Geometry: final body of the model. Coordinates: model frame, mm. A direction names the side the tool comes from. Coordinates: 2 decimals unless noted, no trailing zeros. Order: outer loops, then holes, each group sorted by start corner. A loop starts at its lowest first (then second) coordinate and runs counter-clockwise, first axis right, second up. Notation, with made-up numbers: M 62.25,57.5 L 83.25,57.5 A18 cw 83.25,61.5 Z; hole C 69,-9.5 d7. An arc over 180 degrees is marked long. Write item = value, one per line. Start each with the question number.
```python
from build123d import *

# Parameters (mm, degrees)
ESQUISSE1_W             = 50
ESQUISSE1_H             = 17
BOSS_EXTRU_1_DEPTH      = 35
D_POUILLE2_ANGLE        = -5
COQUE2_T                = -1
CONG_1_R                = 1
ESQUISSE2_R             = 2
ESQUISSE2_R_2           = 1
BOSS_EXTRU_2_DEPTH      = 14.5
ENL_V_MAT_EXTRU_1_REACH = 48.249
ENL_V_MAT_EXTRU_2_REACH = 48.249
ESQUISSE4_R             = 1.5


with BuildPart() as part:
    # Esquisse1 → Boss.-Extru.1 (new body)
    with BuildSketch(Plane.XY):
        with Locations((0, 8.5)):
            Rectangle(ESQUISSE1_W, ESQUISSE1_H)
    extrude(amount=BOSS_EXTRU_1_DEPTH)

    # Dépouille2
    d_pouille2_faces = [part.faces().sort_by_distance(p)[0] for p in [
        (0, 8.5, 0),
        (25, 8.5, 17.5),
        (-25, 8.5, 17.5),
        (0, 8.5, 35),
    ]]
    draft(d_pouille2_faces, Plane(origin=(-25, 0, 35), x_dir=(-1, 0, 0), z_dir=(0, -1, 0)), D_POUILLE2_ANGLE)

    # Coque2
    coque2_openings = [part.faces().sort_by_distance(p)[0] for p in [
        (0, 0, 17.5),
    ]]
    offset(amount=COQUE2_T, openings=coque2_openings, kind=Kind.INTERSECTION)

    # Congé1
    cong_1_edges = [part.edges().sort_by_distance(p)[0] for p in [
        (24.25634636, 8.5, 34.25634636),
        (0, 17, 33.51269272),
        (-23.296270854, 8, 1.703729146),
        (-22.596361546, 16, 17.5),
        (23.296270854, 8, 1.703729146),
        (0, 16, 2.403638454),
        (22.596361546, 16, 17.5),
        (-23.296270854, 8, 33.296270854),
        (23.296270854, 8, 33.296270854),
        (0, 16, 32.596361546),
        (-24.25634636, 8.5, 34.25634636),
        (0, 17, 1.48730728),
        (24.25634636, 8.5, 0.74365364),
        (-24.25634636, 8.5, 0.74365364),
        (-23.51269272, 17, 17.5),
        (23.51269272, 17, 17.5),
    ]]
    fillet(cong_1_edges, radius=CONG_1_R)

    # Esquisse2 → Boss.-Extru.2 (add)
    # profile 1 of 2: a face of its own
    with BuildSketch(Plane(origin=(0, 16, 0), x_dir=(-1, 0, 0), z_dir=(0, -1, 0))):
        with Locations(Location((-19.25, -29.25, 0), (0, 0, 270))):
            Circle(ESQUISSE2_R)
        with Locations(Location((-19.25, -29.25, 0), (0, 0, 270))):
            Circle(ESQUISSE2_R_2, mode=Mode.SUBTRACT)
    # profile 2 of 2: a face of its own
    with BuildSketch(Plane(origin=(0, 16, 0), x_dir=(-1, 0, 0), z_dir=(0, -1, 0))):
        with Locations(Location((19.25, -5.75, 0), (0, 0, 270))):
            Circle(ESQUISSE2_R)
        with Locations(Location((19.25, -5.75, 0), (0, 0, 270))):
            Circle(ESQUISSE2_R_2, mode=Mode.SUBTRACT)
    extrude(amount=BOSS_EXTRU_2_DEPTH)

    # Esquisse3 → Enlèv. mat.-Extru.1 (cut, up to next)
    with BuildSketch(Plane(origin=(0, 0, 0), x_dir=(0, 0, -1), z_dir=(1, 0, 0)), mode=Mode.PRIVATE) as enl_v_mat_extru_1_sk1:
        with BuildLine():
            Line((-20, 5), (-20, -1))
            Line((-20, -1), (-15, -1))
            Line((-15, -1), (-15, 5))
            ThreePointArc((-15, 5), (-17.5, 7.5), (-20, 5))
        make_face()
    enl_v_mat_extru_1_tool1 = extrude(enl_v_mat_extru_1_sk1.sketch, amount=-ENL_V_MAT_EXTRU_1_REACH, mode=Mode.PRIVATE) & part.part
    add(enl_v_mat_extru_1_tool1.solids().sort_by_distance((0, 3.001296, 17.5))[0], mode=Mode.SUBTRACT)

    # Enlèv. mat.-Extru.2: up to this plane
    enl_v_mat_extru_2_end = Plane(origin=(25, 0, 35), z_dir=(0.9961946980917455, 0.08715574274765836, 0))
    # Esquisse4 → Enlèv. mat.-Extru.2 (cut, up to the surface)
    with BuildSketch(Plane(origin=(0, 0, 0), x_dir=(0, 0, -1), z_dir=(1, 0, 0)), mode=Mode.PRIVATE) as enl_v_mat_extru_2_sk1:
        with Locations(Location((-8, 6, 0), (0, 0, 90))):
            Circle(ESQUISSE4_R)
    enl_v_mat_extru_2_tool1 = split(extrude(enl_v_mat_extru_2_sk1.sketch, amount=ENL_V_MAT_EXTRU_2_REACH, mode=Mode.PRIVATE), bisect_by=enl_v_mat_extru_2_end, keep=Keep.BOTH, mode=Mode.PRIVATE)
    add(enl_v_mat_extru_2_tool1.solids().sort_by_distance((0, 6, 8))[0], mode=Mode.SUBTRACT)


solid = part.part
```
Item 1: First-contact query: pin 1 (10 mm diameter, centred on x = 2, y = 15, fed in from +Z); pin 2 (10 mm diameter, centred on x = 17.5, y = 8.5, fed in from +Z); pin 3 (4 mm diameter, centred on y = 12, z = 31, fed in from -X). Flat tips, straight axial feed; report the tip coordinate or a pass-through.
Item 2: Reachability of faces 1 (the flat face through (23.345, 7.438, 17.283)), 2 (the cylindrical face through (0.316, 16.744, 33.264)), 3 (the cylindrical face through (-23.9, 7.5, 17.4)) from +Z, -Z, +X, -X, +Y, -Y: full face, straight path, thin tool, end or side. Return the list, or none.
Item 3: Section query B-B on x = 19.25. Output: boundary loops of the cut face in (y, z), and give its area (3 significant figures).
Item 4: Draft query along Z for faces 4 (the cylindrical face through (-24, 8.17, 33.99)), 5 (the cylindrical face through (0.316, 16.744, 1.736)), 6 (the flat face through (20, 1.5, 28)), 7 (the flat face through (-24.306, 7.931, 17.269)). Return one class per face: pulls with the +Z half, pulls with the -Z half, needs draft (parallel to the pull), parting line crosses it, or undercut.
Item 5: Section query A-A on z = 22.5. Output: boundary loops of the cut face in (x, y), and give its area (3 significant figures).
Item 6: Material intervals for probe 1 along Z at (x, y) = (18.5, 14.25); probe 2 along X at (y, z) = (7, 29.25); probe 3 along X at (y, z) = (2.75, 4.5), sorted ascending. Write a range as [from, to].
Item 7: Section query D-D on x = 6.5. Output: boundary loops of the cut face in (y, z), and give its area (3 significant figures).
Item 8: Section query C-C on y = 12.5. Give the number of separate pieces and of enclosed holes in the cut face, and give its area (3 significant figures).
Ans:
q1.pin_1 = 34.13
q1.pin_2 = 34.69
q1.pin_3 = -24.13
q2.face_1 = -Y
q2.face_2 = +Z, +X, -X, +Y
q2.face_3 = -X, -Y
q3.outline = M 0,0 L 16.09,1.41 A1 ccw 17,2.4 L 17,32.6 A1 ccw 16.09,33.59 L 0,35 L 0,34 L 15.09,32.68 A1 cw 16,31.68 L 16,31.25 L 1.5,31.25 L 1.5,30.25 L 16,30.25 L 16,28.25 L 1.5,28.25 L 1.5,27.25 L 16,27.25 L 16,3.32 A1 cw 15.09,2.32 L 0,1 Z
q3.area = 93.2 mm^2
q4.face_4 = pulls with the +Z half
q4.face_5 = pulls with the -Z half
q4.face_6 = undercut
q4.face_7 = needs draft
q5.outline = M -25,0 L -24,0 L -22.68,15.09 A1 cw -21.68,16 L 21.68,16 A1 cw 22.68,15.09 L 24,0 L 25,0 L 23.59,16.09 A1 ccw 22.6,17 L -22.6,17 A1 ccw -23.59,16.09 Z
q5.area = 79.2 mm^2
q6.probe_1 = [1.25, 2.25], [27.4, 28.59], [29.91, 31.1], [32.75, 33.75]
q6.probe_2 = [-24.39, -23.38], [17.25, 18.25], [20.25, 21.25], [23.38, 24.39]
q6.probe_3 = [-24.76, -23.76], [-20.81, -17.69], [23.76, 24.76]
q7.outline = M 0,0 L 16.09,1.41 A1 ccw 17,2.4 L 17,32.6 A1 ccw 16.09,33.59 L 0,35 L 0,34 L 15.09,32.68 A1 cw 16,31.68 L 16,3.32 A1 cw 15.09,2.32 L 0,1 Z
q7.area = 64.2 mm^2
q8.separate_pieces = 3
q8.enclosed_holes = 3
q8.area = 177 mm^2
